```python
from build123d import *

# Parameters (mm, degrees)
SKETCH_W     = 60
SKETCH_H     = 35
PAD_DEPTH    = 20
FILLET_R     = 5
THICKNESS_T  = -1.5
SKETCH001_W  = 5
SKETCH001_H  = 8
SKETCH001_R  = 1.5
PAD001_DEPTH = 5
FILLET001_R  = 2.49


with BuildPart() as part:
    # Sketch → Pad (new body)
    with BuildSketch(Plane.XY):
        Rectangle(SKETCH_W, SKETCH_H)
    extrude(amount=-PAD_DEPTH)

    # Fillet
    fillet_edges = [part.edges().sort_by_distance(p)[0] for p in [
        (0, -17.5, -20),
        (30, 0, -20),
        (0, 17.5, -20),
        (-30, 0, -20),
        (30, 17.5, -10),
        (30, -17.5, -10),
        (-30, 17.5, -10),
        (-30, -17.5, -10),
    ]]
    fillet(fillet_edges, radius=FILLET_R)

    # Thickness
    thickness_openings = [part.faces().sort_by_distance(p)[0] for p in [
        (0, 0, 0),
    ]]
    offset(amount=THICKNESS_T, openings=thickness_openings)

    # Sketch001 → Pad001 (join, symmetric)
    with BuildSketch(Plane.YZ):
        with Locations((20, 1)):
            Rectangle(SKETCH001_W, SKETCH001_H)
        with Locations((20, 2.5)):
            Circle(SKETCH001_R, mode=Mode.SUBTRACT)
    extrude(amount=PAD001_DEPTH, both=True)

    # Fillet001
    fillet001_edges = [part.edges().sort_by_distance(p)[0] for p in [
        (0, 22.5, 5),
        (0, 17.5, 5),
        (0, 22.5, -3),
    ]]
    fillet(fillet001_edges, radius=FILLET001_R)


solid = part.part
```
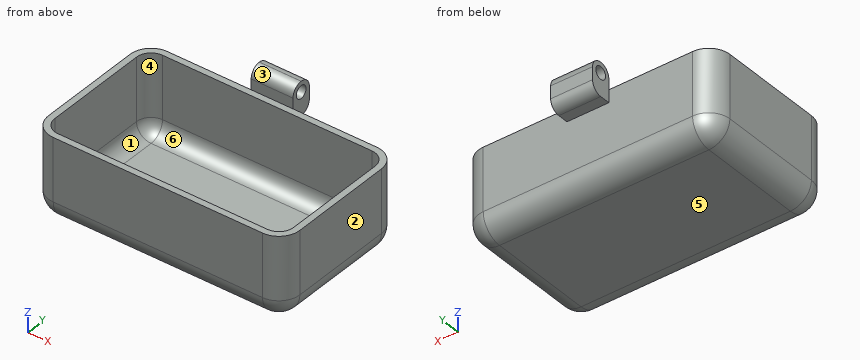
Could you check a few things on this model? Use its own coordinates, in mm. Face numbers are marked on the shaded views. A direction names the side the tool comes from. Coordinates: 2 decimals unless noted, no trailing zeros. Write each loop counter-clockwise with the first axis right and the second up, starting at its lowest first coordinate (ties: lowest second). Pieces come first, ordered by that corner, then holes. Notation, with made-up numbers: (14.25, 67.5) -> (68.25, 67.5) arc R10 cw to (68.25, 75.5) -> close; hole circle Ø9 at (-32, 18). An arc over 180 degrees is marked (long way). Return JSON: item names as keys, results as strings.
(1) Which directions (+Z, -Z, +X, -X, +Y, -Y) give clear straight access to the entire face, cutting with the end or side of a thin tool? Please do the marked faces 5 and 6.
Numbers:
{"face 5": "-Z, +X, -X, +Y, -Y", "face 6": "+Z"}
(2) I need wall thicknesses on L1, parallel to X at y = -3, z = -13.25; L2, parallel to Z at x = -0.5, y = 20; L3, parallel to Y at x = -20, z = -0.5. Which ranges of each line are inside material? Lowest first, please.
Numbers:
{"L1": "x = -30 to -28.5, 28.5 to 30", "L2": "z = -3 to 1, 4 to 5", "L3": "y = -17.5 to -16, 16 to 17.5"}
(3) Imagine slicing it at B-B, the plane z = -14. Please give me the cut outline in (x, y).
Numbers:
{"outline": "(-30, -12.5) arc R5 ccw to (-25, -17.5) -> (25, -17.5) arc R5 ccw to (30, -12.5) -> (30, 12.5) arc R5 ccw to (25, 17.5) -> (-25, 17.5) arc R5 ccw to (-30, 12.5) -> close; hole (-28.5, -12.5) arc R3.5 ccw to (-25, -16) -> (25, -16) arc R3.5 ccw to (28.5, -12.5) -> (28.5, 12.5) arc R3.5 ccw to (25, 16) -> (-25, 16) arc R3.5 ccw to (-28.5, 12.5) -> close"}
(4) I'm going to push flat-ended pins straight in: pin 1 (4 mm diameter, centred on x = 14.5, z = 0.5, fed in from +Y); pin 2 (1.5 mm diameter, centred on y = 19, z = -0.5, fed in from -X); pin 3 (12.5 mm diameter, centred on x = -9.5, y = 6, fed in from +Z); pin 4 (1.8 mm diameter, centred on y = 20, z = 2.5, fed in from +X). Where does each tip first touch, or does it pass through?
Numbers:
{"pin 1": "stops at y = 17.5", "pin 2": "stops at x = -5", "pin 3": "stops at z = -18.5", "pin 4": "passes through"}
(5) Imagine slicing it at D-D, the plane z = -2. Please give me the cut outline in (x, y) (3 decimals), then the cut area to 3 significant figures.
Numbers:
{"outline": "(-30, -12.5) arc R5 ccw to (-25, -17.5) -> (25, -17.5) arc R5 ccw to (30, -12.5) -> (30, 12.5) arc R5 ccw to (25, 17.5) -> (5, 17.5) -> (5, 22.005) -> (-5, 22.005) -> (-5, 17.5) -> (-25, 17.5) arc R5 ccw to (-30, 12.5) -> close; hole (-28.5, -12.5) arc R3.5 ccw to (-25, -16) -> (25, -16) arc R3.5 ccw to (28.5, -12.5) -> (28.5, 12.5) arc R3.5 ccw to (25, 16) -> (-25, 16) arc R3.5 ccw to (-28.5, 12.5) -> close", "area": "310 mm2"}
(6) Imagine slicing it at A-A, the plane y = -7.5. Please give me the cut outline in (x, z), then the cut area to 3 significant figures.
Numbers:
{"outline": "(-30, -15) arc R5 ccw to (-25, -20) -> (25, -20) arc R5 ccw to (30, -15) -> (30, 0) -> (28.5, 0) -> (28.5, -15) arc R3.5 cw to (25, -18.5) -> (-25, -18.5) arc R3.5 cw to (-28.5, -15) -> (-28.5, 0) -> (-30, 0) -> close", "area": "140 mm2"}
(7) Imagine slicing it at C-C, the plane x = 17. Please give me the cut outline in (y, z), then the cut area to 3 significant figures.
Numbers:
{"outline": "(-17.5, -15) arc R5 ccw to (-12.5, -20) -> (12.5, -20) arc R5 ccw to (17.5, -15) -> (17.5, 0) -> (16, 0) -> (16, -15) arc R3.5 cw to (12.5, -18.5) -> (-12.5, -18.5) arc R3.5 cw to (-16, -15) -> (-16, 0) -> (-17.5, 0) -> close", "area": "103 mm2"}
(8) We'd pull the mould along Y, two halves only. Please class the marked faces 1, 2, 3 and 4: +Y half, -Y half, draft (parallel to the pull), parting line (faces both ways), or undercut.
Numbers:
{"face 1": "undercut", "face 2": "draft", "face 3": "-Y half", "face 4": "undercut"}
